```python
from build123d import *

# Parameters (mm, degrees)
ESTRUSIONE_ESTRUSIONE1_DEPTH = 18
TAGLIO_ESTRUSIONE1_DEPTH     = 115
TAGLIO_ESTRUSIONE2_DEPTH     = 258
TAGLIO_ESTRUSIONE3_DEPTH     = 723
TAGLIO_ESTRUSIONE4_DEPTH     = 160
TAGLIO_ESTRUSIONE5_DEPTH     = 190
TAGLIO_ESTRUSIONE6_DEPTH     = 231


with BuildPart() as part:
    # Schizzo2 → Estrusione-Estrusione1 (new body)
    with BuildSketch(Plane.XY):
        with BuildLine():
            Line((-275, -250), (-275, -214))
            Line((-275, -214), (-257, -214))
            ThreePointArc((-257, -214), (-253.825, -210.825), (-257, -207.65))
            Line((-257, -207.65), (-257, -180.35))
            ThreePointArc((-257, -180.35), (-253.825, -177.175), (-257, -174))
            Line((-257, -174), (-275, -174))
            Line((-275, -174), (-275, 174))
            Line((-275, 174), (-257, 174))
            ThreePointArc((-257, 174), (-253.825, 177.175), (-257, 180.35))
            Line((-257, 180.35), (-257, 207.65))
            ThreePointArc((-257, 207.65), (-253.825, 210.825), (-257, 214))
            Line((-257, 214), (-275, 214))
            Line((-275, 214), (-275, 250))
            Line((-275, 250), (-225, 250))
            Line((-225, 250), (-225, 232))
            ThreePointArc((-225, 232), (-221.825, 228.825), (-218.65, 232))
            Line((-218.65, 232), (-181.35, 232))
            ThreePointArc((-181.35, 232), (-178.175, 228.825), (-175, 232))
            Line((-175, 232), (-175, 250))
            Line((-175, 250), (-125, 250))
            Line((-125, 250), (-125, 232))
            ThreePointArc((-125, 232), (-121.825, 228.825), (-118.65, 232))
            Line((-118.65, 232), (-81.35, 232))
            ThreePointArc((-81.35, 232), (-78.175, 228.825), (-75, 232))
            Line((-75, 232), (-75, 250))
            Line((-75, 250), (-25, 250))
            Line((-25, 250), (-25, 232))
            ThreePointArc((-25, 232), (-21.825, 228.825), (-18.65, 232))
            Line((-18.65, 232), (18.65, 232))
            ThreePointArc((18.65, 232), (21.825, 228.825), (25, 232))
            Line((25, 232), (25, 250))
            Line((25, 250), (75, 250))
            Line((75, 250), (75, 232))
            ThreePointArc((75, 232), (78.175, 228.825), (81.35, 232))
            Line((81.35, 232), (118.65, 232))
            ThreePointArc((118.65, 232), (121.825, 228.825), (125, 232))
            Line((125, 232), (125, 250))
            Line((125, 250), (175, 250))
            Line((175, 250), (175, 232))
            ThreePointArc((175, 232), (178.175, 228.825), (181.35, 232))
            Line((181.35, 232), (218.65, 232))
            ThreePointArc((218.65, 232), (221.825, 228.825), (225, 232))
            Line((225, 232), (225, 250))
            Line((225, 250), (275, 250))
            Line((275, 250), (275, -250))
            Line((275, -250), (225, -250))
            Line((225, -250), (225, -232))
            ThreePointArc((225, -232), (221.825, -228.825), (218.65, -232))
            Line((218.65, -232), (181.35, -232))
            ThreePointArc((181.35, -232), (178.175, -228.825), (175, -232))
            Line((175, -232), (175, -250))
            Line((175, -250), (125, -250))
            Line((125, -250), (125, -232))
            ThreePointArc((125, -232), (121.825, -228.825), (118.65, -232))
            Line((118.65, -232), (81.35, -232))
            ThreePointArc((81.35, -232), (78.175, -228.825), (75, -232))
            Line((75, -232), (75, -250))
            Line((75, -250), (25, -250))
            Line((25, -250), (25, -232))
            ThreePointArc((25, -232), (21.825, -228.825), (18.65, -232))
            Line((18.65, -232), (-18.65, -232))
            ThreePointArc((-18.65, -232), (-21.825, -228.825), (-25, -232))
            Line((-25, -232), (-25, -250))
            Line((-25, -250), (-75, -250))
            Line((-75, -250), (-75, -232))
            ThreePointArc((-75, -232), (-78.175, -228.825), (-81.35, -232))
            Line((-81.35, -232), (-118.65, -232))
            ThreePointArc((-118.65, -232), (-121.825, -228.825), (-125, -232))
            Line((-125, -232), (-125, -250))
            Line((-125, -250), (-175, -250))
            Line((-175, -250), (-175, -232))
            ThreePointArc((-175, -232), (-178.175, -228.825), (-181.35, -232))
            Line((-181.35, -232), (-218.65, -232))
            ThreePointArc((-218.65, -232), (-221.825, -228.825), (-225, -232))
            Line((-225, -232), (-225, -250))
            Line((-225, -250), (-275, -250))
        make_face()
    extrude(amount=ESTRUSIONE_ESTRUSIONE1_DEPTH)

    # Schizzo2<4> → Taglio-Estrusione1 (cut)
    with BuildSketch(Plane.XY):
        with BuildLine():
            Line((237, 145.65), (237, 108.35))
            ThreePointArc((237, 108.35), (233.825, 105.175), (237, 102))
            Line((237, 102), (255, 102))
            ThreePointArc((255, 102), (258.175, 105.175), (255, 108.35))
            Line((255, 108.35), (255, 145.65))
            ThreePointArc((255, 145.65), (258.175, 148.825), (255, 152))
            Line((255, 152), (237, 152))
            ThreePointArc((237, 152), (233.825, 148.825), (237, 145.65))
        make_face()
    extrude(amount=TAGLIO_ESTRUSIONE1_DEPTH, mode=Mode.SUBTRACT)

    # Schizzo2<5> → Taglio-Estrusione2 (cut)
    with BuildSketch(Plane.XY):
        with BuildLine():
            Line((255, -18.65), (255, 18.65))
            ThreePointArc((255, 18.65), (258.175, 21.825), (255, 25))
            Line((255, 25), (237, 25))
            ThreePointArc((237, 25), (233.825, 21.825), (237, 18.65))
            Line((237, 18.65), (237, -18.65))
            ThreePointArc((237, -18.65), (233.825, -21.825), (237, -25))
            Line((237, -25), (255, -25))
            ThreePointArc((255, -25), (258.175, -21.825), (255, -18.65))
        make_face()
    extrude(amount=TAGLIO_ESTRUSIONE2_DEPTH, mode=Mode.SUBTRACT)

    # Schizzo2<7> → Taglio-Estrusione3 (cut)
    with BuildSketch(Plane.XY):
        with BuildLine():
            Line((255, -152), (237, -152))
            ThreePointArc((237, -152), (233.825, -148.825), (237, -145.65))
            Line((237, -145.65), (237, -108.35))
            ThreePointArc((237, -108.35), (233.825, -105.175), (237, -102))
            Line((237, -102), (255, -102))
            ThreePointArc((255, -102), (258.175, -105.175), (255, -108.35))
            Line((255, -108.35), (255, -145.65))
            ThreePointArc((255, -145.65), (258.175, -148.825), (255, -152))
        make_face()
    extrude(amount=TAGLIO_ESTRUSIONE3_DEPTH, mode=Mode.SUBTRACT)

    # Schizzo2<8> → Taglio-Estrusione4 (cut)
    with BuildSketch(Plane.XY):
        with BuildLine():
            Line((-255, 152), (-237, 152))
            ThreePointArc((-237, 152), (-233.825, 148.825), (-237, 145.65))
            Line((-237, 145.65), (-237, 108.35))
            ThreePointArc((-237, 108.35), (-233.825, 105.175), (-237, 102))
            Line((-237, 102), (-255, 102))
            ThreePointArc((-255, 102), (-258.175, 105.175), (-255, 108.35))
            Line((-255, 108.35), (-255, 145.65))
            ThreePointArc((-255, 145.65), (-258.175, 148.825), (-255, 152))
        make_face()
    extrude(amount=TAGLIO_ESTRUSIONE4_DEPTH, mode=Mode.SUBTRACT)

    # Schizzo2<9> → Taglio-Estrusione5 (cut)
    with BuildSketch(Plane.XY):
        with BuildLine():
            Line((-255, 25), (-237, 25))
            ThreePointArc((-237, 25), (-233.825, 21.825), (-237, 18.65))
            Line((-237, 18.65), (-237, -18.65))
            ThreePointArc((-237, -18.65), (-233.825, -21.825), (-237, -25))
            Line((-237, -25), (-255, -25))
            ThreePointArc((-255, -25), (-258.175, -21.825), (-255, -18.65))
            Line((-255, -18.65), (-255, 18.65))
            ThreePointArc((-255, 18.65), (-258.175, 21.825), (-255, 25))
        make_face()
    extrude(amount=TAGLIO_ESTRUSIONE5_DEPTH, mode=Mode.SUBTRACT)

    # Schizzo2<10> → Taglio-Estrusione6 (cut)
    with BuildSketch(Plane.XY):
        with BuildLine():
            Line((-237, -145.65), (-237, -108.35))
            ThreePointArc((-237, -108.35), (-233.825, -105.175), (-237, -102))
            Line((-237, -102), (-255, -102))
            ThreePointArc((-255, -102), (-258.175, -105.175), (-255, -108.35))
            Line((-255, -108.35), (-255, -145.65))
            ThreePointArc((-255, -145.65), (-258.175, -148.825), (-255, -152))
            Line((-255, -152), (-237, -152))
            ThreePointArc((-237, -152), (-233.825, -148.825), (-237, -145.65))
        make_face()
    extrude(amount=TAGLIO_ESTRUSIONE6_DEPTH, mode=Mode.SUBTRACT)


solid = part.part
```
The model under review builds one solid part; all positions refer to its coordinate system, in mm. A direction names the side the tool comes from. Round coordinates to 2 decimals unless told otherwise and drop trailing zeros. Write each loop counter-clockwise with the first axis right and the second up, starting at its lowest first coordinate (ties: lowest second). Pieces come first, ordered by that corner, then holes.
(1) Insertion check: pin 1 (5 mm diameter, centred on x = -81, z = 12, fed in from -Y); pin 2 (5.5 mm diameter, centred on y = -192, z = 6, fed in from -X); pin 3 (5.5 mm diameter, centred on x = -104.5, z = 6.5, fed in from +Y). Each pin has a flat end and moves straight along its axis. Give the tip position at first contact, or say it passes through.
(2) We need section B-B on z = 3.5. Give the number of separate pieces and of enclosed holes in the cut face, and give its area (3 significant figures).
(3) Wall thickness on L1, parallel to X at y = -117, z = 6.5; L2, parallel to X at y = 22.5, z = 16; L3, parallel to Y at x = -205, z = 17: over which ranges is each line inside the solid? List them lowest first.
(4) We need section A-A on y = 3.5. Give the boundary of the cut face in (x, z), and give its area (3 significant figures).
(5) Mouldability with a two-part tool opening along Y and no side actions: class faces 6 (the flat face through (-266, 214, 9)), 7 (the flat face through (-225, 241, 9)), 8 (the flat face through (-50, -250, 9)) as +Y half, -Y half, draft (parallel to the pull), parting line (faces both ways), or undercut.
(6) Machinability: for faces 1 (the flat face through (100, -232, 9)), 2 (the flat face through (-250, 250, 9)), 3 (the flat face through (-200, 232, 9)), 4 (the flat face through (237, 0, 9)), 5 (the flat face through (275, 3, 9)), which of the approach directions +Z, -Z, +X, -X, +Y, -Y give a long, thin tool a straight path to every point of the face, cutting with its end or side? Answer none if there is none.
Findings below:
1. pin 1: stops at y = -232
1. pin 2: stops at x = -257
1. pin 3: stops at y = 232
2. separate pieces: 1
2. enclosed holes: 6
2. area: 258,000 mm2
3. L1: x = -275 to -255, -237 to 237, 255 to 275
3. L2: x = -275 to -258.1, -233.9 to 233.9, 258.1 to 275
3. L3: y = -232 to 232
4. outline: (-275, 0) - (-255, 0) - (-255, 18) - (-275, 18) - close; (-237, 0) - (237, 0) - (237, 18) - (-237, 18) - close; (255, 0) - (275, 0) - (275, 18) - (255, 18) - close
4. area: 9,250 mm2
5. face 6: undercut
5. face 7: draft
5. face 8: -Y half
6. face 1: +Z, -Z, -Y
6. face 2: +Z, -Z, +X, -X, +Y
6. face 3: +Z, -Z, +Y
6. face 4: +Z, -Z
6. face 5: +Z, -Z, +X, +Y, -Y
